Autodesk Fusion 360 part; units mm, degrees
sketch "Sketch1" plane through (0, 0, 0) normal (0, 1, 0) x (1, 0, 0)
  line L0 (-39.5, 0) -> (-39.5, 6)
  line L1 (-39.5, 6) -> (-22.8391, 6)
  line L2 (-50, 0) -> (42, 0) construction
  line L3 (0, 0) -> (18.7964, 26.8441) construction
  arc A0 (9.38, 13.9978) -> (-16.85, 0) centre (0, 0) ccw
  arc A1 (12.8944, 15.7435) -> (-18.3343, 8.8304) centre (0, 0) ccw
  arc A2 (-22.8391, 6) -> (-18.3343, 8.8304) centre (-22.8391, 11) ccw
  line L4 (-28.5277, 8) -> (-28.5277, 0)
  line L5 (-39.5, -6) -> (-22.8391, -6)
  arc A3 (-18.3343, -8.8304) -> (-22.8391, -6) centre (-22.8391, -11) ccw
  line L6 (-28.5277, -8) -> (-28.5277, 0)
  arc A4 (-16.85, 0) -> (9.38, -13.9978) centre (0, 0) ccw
  line L7 (-39.5, 0) -> (-39.5, -6)
  arc A5 (9.8515, 13.8322) -> (12.4661, 13.9912) centre (10.6183, 22.7994) ccw
  line L8 (0, 28) -> (0, 20.2823) construction
  line L9 (0, 20.35) -> (0, -24) construction
  arc A6 (12.4661, 13.9912) -> (12.8944, 15.7435) centre (12.2608, 14.9699) ccw
  arc A7 (9.38, 13.9978) -> (9.8515, 13.8322) centre (9.9367, 14.8285) ccw
  arc A8 (12.8944, -15.7435) -> (12.4661, -13.9912) centre (12.2608, -14.9699) ccw
  arc A9 (12.4661, -13.9912) -> (9.8515, -13.8322) centre (10.6183, -22.7994) ccw
  arc A10 (9.8515, -13.8322) -> (9.38, -13.9978) centre (9.9367, -14.8285) ccw
  line L10 (-0.661, 0) -> (-0.661, -36.4532) construction
  line L11 (3.815, 0) -> (3.815, -36.4532) construction
  line L12 (-0.661, -36.4532) -> (3.815, -36.4532) construction
  line L13 (-0.073, -19.5) -> (-0.073, -20.3)
  line L14 (-0.073, -20.3) -> (3.227, -20.3)
  line L15 (3.227, -19.5) -> (3.227, -20.3)
  arc A11 (3.227, -19.5) -> (-0.073, -19.5) centre (1.577, -19.5) ccw
  line L16 (-0.073, -20.3) -> (-13.423, -20.3)
  line L17 (-13.423, -20.3) -> (-13.423, -30.3)
  line L18 (-13.423, -30.3) -> (-16.923, -30.3)
  line L19 (-5.423, -20.3) -> (-5.423, -11) construction
  arc A12 (-18.3343, -8.8304) -> (-1.4257, -20.3) centre (0, 0) ccw
  arc A13 (1.4257, -20.3) -> (12.8944, -15.7435) centre (0, 0) ccw
  line L20 (-0.073, -22.3) -> (-11.423, -22.3)
  line L21 (-11.423, -22.3) -> (-11.423, -30.3)
  line L22 (-11.423, -30.3) -> (-13.423, -30.3)
  line L23 (-0.073, -22.3) -> (-0.073, -20.3)
  line L24 (-0.073, -20.3) -> (-0.073, -16.8498)
  line L25 (3.227, -20.3) -> (3.227, -16.5381)
  line L26 (-16.923, -30.3) -> (-16.923, -11.302)
  line L27 (-22.8391, -6) -> (-22.8391, 6)
  line L28 (-20.179, -6.7663) -> (-20.179, 6.7663)
  point P0 (-50, 0)
  dimension "d1" = 33.7
  dimension "d4" = 6
  dimension "d5" = 39.5
  dimension "d6" = 3.5
  dimension "d7" = 5
  dimension "d11" = 55
  dimension "d30" = 1
  dimension "d31" = 9
  dimension "d32" = 1
  dimension "d36" = 3.815
  dimension "d37" = 3.3
  dimension "d39" = 0.661
  dimension "d40" = 4.476
  dimension "d41" = 2.238
  dimension "d42" = 0.8
  dimension "d43" = 19.5
  dimension "d44" = 15
  dimension "d45" = 7
  dimension "d46" = 10
  dimension "d47" = 3.5
  dimension "d48" = -2
  dimension "d70" = 28.5277
extrude "Extrude1" add sketch "Sketch1" along normal mid plane 10 contours A2 A3 L27 L28 | A0 A1 A2 A3 A4 A5 A6 A7 L13 L16 A12 L24 L28 | L13 L14 L15 A11 A13 L24 L25 | A4 A11 L24 L25 | A4 A8 A9 A10 L15 A13 L25
ref_plane "WorkPlane1" through (-16.85, 0, 0) normal (1, 0, 0) x (0, 1, 0)
sketch "Sketch2" plane through (-16.85, 0, 0) normal (1, 0, 0) x (0, 0, -1)
  line L0 (-1.6743, 2.9) -> (-3.3486, 0)
  line L1 (-3.3486, 0) -> (-1.6743, -2.9)
  line L2 (-1.6743, -2.9) -> (1.6743, -2.9)
  line L3 (1.6743, -2.9) -> (3.3486, 0)
  line L4 (3.3486, 0) -> (1.6743, 2.9)
  line L5 (1.6743, 2.9) -> (-1.6743, 2.9)
  circle A0 centre (0, 0) radius 1.6
  line L6 (-1.175, 2.175) -> (1.175, 2.175)
  line L7 (2.175, 1.175) -> (2.175, -1.175)
  line L8 (1.175, -2.175) -> (-1.175, -2.175)
  line L9 (-2.175, -1.175) -> (-2.175, 1.175)
  line L10 (-2.175, 2.175) -> (2.175, -2.175) construction
  line L11 (2.175, 2.175) -> (-2.175, -2.175) construction
  arc A1 (-1.175, 2.175) -> (-2.175, 1.175) centre (-1.175, 1.175) ccw
  arc A2 (-2.175, -1.175) -> (-1.175, -2.175) centre (-1.175, -1.175) ccw
  arc A3 (1.175, -2.175) -> (2.175, -1.175) centre (1.175, -1.175) ccw
  arc A4 (2.175, 1.175) -> (1.175, 2.175) centre (1.175, 1.175) ccw
  circle A5 centre (0, 2.175) radius 2.25
  dimension "d16" = 2.9
  dimension "d104" = 4.35
  dimension "d105" = 4.35
  dimension "d106" = 1
  dimension "d125" = 4.5
ref_plane "WorkPlane2" through (0, 4.9, 0) normal (0, 1, 0) x (0, 0, 1)
extrude "Extrude19" add sketch "Sketch1" along normal blind 8.3 contours A2 A3 L27 L28
sketch "Sketch11" plane through (0, 8.3, 0) normal (0, 1, 0) x (-1, 0, 0)
  arc A0 (20.179, 6.7663) -> (22.8391, 6) centre (22.8391, 11) ccw
  line L0 (20.179, 6.7663) -> (20.179, -6.7663)
  arc A1 (22.8391, -6) -> (20.179, -6.7663) centre (22.8391, -11) ccw
  line L1 (22.8391, -6) -> (22.8391, 6)
  line L2 (22.8391, -29.79) -> (-66.1609, -29.79)
  line L3 (-66.1609, -29.79) -> (-66.1609, 29.79)
  line L4 (-66.1609, 29.79) -> (22.8391, 29.79)
  line L5 (22.8391, 29.79) -> (22.8391, -29.79)
  line L6 (22.8391, 6) -> (22.8391, -6)
  point P0 (22.8391, -6)
  dimension "d116" = 89
  dimension "d117" = 59.58
  dimension "d118" = 29.79
extrude "Extrude20" add sketch "Sketch11" along normal blind 1.83
sketch "Sketch12" plane through (0, -5, 0) normal (0, -1, 0) x (1, 0, 0)
  arc A0 (-1.4257, 20.3) -> (-18.3343, 8.8304) centre (0, 0) ccw
  arc A1 (-22.8391, 6) -> (-18.3343, 8.8304) centre (-22.8391, 11) ccw
  line L0 (-22.8391, 6) -> (-22.8391, -6)
  arc A2 (-18.3343, -8.8304) -> (-22.8391, -6) centre (-22.8391, -11) ccw
  arc A3 (-18.3343, -8.8304) -> (12.8944, -15.7435) centre (0, 0) ccw
  arc A4 (12.8944, -15.7435) -> (12.4661, -13.9912) centre (12.2608, -14.9699) ccw
  arc A5 (12.4661, -13.9912) -> (9.8515, -13.8322) centre (10.6183, -22.7994) ccw
  arc A6 (9.8515, -13.8322) -> (9.38, -13.9978) centre (9.9367, -14.8285) ccw
  arc A7 (9.38, 13.9978) -> (9.38, -13.9978) centre (0, 0) ccw
  arc A8 (9.38, 13.9978) -> (9.8515, 13.8322) centre (9.9367, 14.8285) ccw
  arc A9 (9.8515, 13.8322) -> (12.4661, 13.9912) centre (10.6183, 22.7994) ccw
  arc A10 (12.4661, 13.9912) -> (12.8944, 15.7435) centre (12.2608, 14.9699) ccw
  arc A11 (12.8944, 15.7435) -> (1.4257, 20.3) centre (0, 0) ccw
  line L1 (1.4257, 20.3) -> (-1.4257, 20.3)
  arc A12 (-16.85, 0) -> (9.38, -13.9978) centre (0, 0) ccw
  arc A13 (9.38, 13.9978) -> (-16.85, 0) centre (0, 0) ccw
  circle A14 centre (0, 0) radius 14
  dimension "d128" = 28
extrude "Extrude22" cut sketch "Sketch12" against normal up to surface (15.13 mm away) contours A14
equation "d5 = 50 mm - 10.5 mm"
equation "d41 = ( 4.476 / 2 ) * 1 mm"
equation "d43 = d1 / 2 + 1 mm + d37 / 2"
equation "d114 = 7.4 mm + 0.9 mm"
equation "d118 = d117 / 2"
equation "d120 = 2.23 mm - 0.4 mm"
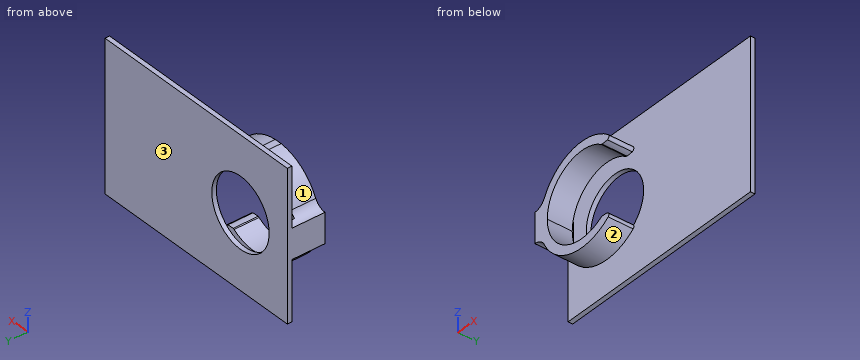
Build history of the part. All positions in model axes, mm. Face numbers are marked on the shaded views. A direction names the side the tool comes from. Round coordinates to 2 decimals unless told otherwise and drop trailing zeros. Loops run counter-clockwise (first coordinate to the right, second up) from the corner with the lowest first, then second, coordinate; pieces in that order, holes last. Notation, with made-up numbers: (37, 60) -> (62, 60) arc R10 ccw to (62, 69) -> close; hole circle Ø7 at (-21, 72.25). An arc over 180 degrees is marked (long way). Use CSV: the item, a comma, the result in double quotes. Start each with the question number.
Q1. Drill centre lines: L1, parallel to Z at x = 0, y = 8.95; L2, parallel to Y at x = 24.5, z = -3.5; L3, parallel to Z at x = -6, y = -2. Where is each one in solid material? Low to high.
Q2. Saw through at B-B on z = 10. Give the cut face in (x, y).
Q3. Saw through at C-C on y = -3.5. Give the cut face in (x, z).
Q4. Flat gauge pins, fed straight in: pin 1 Ø1 at (y, z) = (6.5, 3) entering from +X; pin 2 Ø2 at (y, z) = (3.5, -19.5) entering from -X; pin 3 Ø0.9 at (x, y) = (0, -0.5) entering from +Z. Where does each tip first touch, or does it go through?
Q5. Saw through at A-A on x = 0. Give the cut face in (y, z).
Q6. Which spindle directions (+Z, -Z, +X, -X, +Y, -Y) get a long thin tool onto all of the face, cutting with end or side? Do the marked faces 1, 2 and 3. Say none if no direction does.
Q7. Saw through at D-D on x = -12.5. Give the cut face in (y, z).
Solutions:
1,L1,"z = -29.79 to -14, 14 to 29.79"
1,L2,"y = 8.3 to 10.13"
1,L3,"z = -19.45 to -15.75, 15.75 to 19.45"
2,outline,"(-22.84, 8.3) -> (-9.8, 8.3) -> (-9.8, 10.13) -> (-22.84, 10.13) -> close; (-17.72, -5) -> (-13.56, -5) -> (-13.56, 5) -> (-17.72, 5) -> close; (9.8, 8.3) -> (66.16, 8.3) -> (66.16, 10.13) -> (9.8, 10.13) -> close"
3,outline,"(-22.84, -6) arc R5 cw to (-18.33, -8.83) arc R20.35 ccw to (12.89, -15.74) arc R1 ccw to (12.47, -13.99) arc R9 ccw to (9.85, -13.83) arc R1 ccw to (9.38, -14) arc R16.85 cw to (-16.85, 0) arc R16.85 cw to (9.38, 14) arc R1 ccw to (9.85, 13.83) arc R9 ccw to (12.47, 13.99) arc R1 ccw to (12.89, 15.74) arc R20.35 ccw to (1.43, 20.3) -> (-1.43, 20.3) arc R20.35 ccw to (-18.33, 8.83) arc R5 cw to (-22.84, 6) -> close"
4,pin 1,"stops at x = -20.18"
4,pin 2,"stops at x = -8.48"
4,pin 3,"stops at z = 20.3"
5,outline,"(-5, -20.35) -> (5, -20.35) -> (5, -16.85) -> (-5, -16.85) -> close; (-5, 16.85) -> (5, 16.85) -> (5, 20.3) -> (-5, 20.3) -> close; (8.3, -29.79) -> (10.13, -29.79) -> (10.13, -14) -> (8.3, -14) -> close; (8.3, 14) -> (10.13, 14) -> (10.13, 29.79) -> (8.3, 29.79) -> close"
6,face 1,"+Z, -X, -Y"
6,face 2,"-Z, -Y"
6,face 3,"+Z, -Z, +X, -X, +Y"
7,outline,"(-5, -16.06) -> (5, -16.06) -> (5, -11.3) -> (-5, -11.3) -> close; (-5, 11.3) -> (5, 11.3) -> (5, 16.06) -> (-5, 16.06) -> close; (8.3, -29.79) -> (10.13, -29.79) -> (10.13, -6.3) -> (8.3, -6.3) -> close; (8.3, 6.3) -> (10.13, 6.3) -> (10.13, 29.79) -> (8.3, 29.79) -> close"
